Work out the finished part from the listing and answer in its coordinate system (mm). Round coordinates to 2 decimals unless told otherwise and drop trailing zeros. Order: outer loops, then holes, each group sorted by start corner. A loop starts at its lowest first (then second) coordinate and runs counter-clockwise, first axis right, second up. Notation, with made-up numbers: (74.25, -12.75) - (98.25, -12.75) arc R20 cw to (98.25, 0.25) - close; hole circle Ø6 at (60, 71.25). An arc over 180 degrees is marked (long way). One line per question, with ' | ' between items. Start each with the question number.
from build123d import *

# Parameters (mm, degrees)
SKETCH1_R           = 2.5
SKETCH1_R_2         = 2.7
BOSS_EXTRUDE1_DEPTH = 4
SKETCH4_W           = 280
SKETCH4_H           = 240
SKETCH4_W_2         = 250
SKETCH4_H_2         = 210
CUT_EXTRUDE2_DEPTH  = 10
SKETCH5_R           = 2.5
CUT_EXTRUDE3_DEPTH  = 10


with BuildPart() as part:
    # Sketch1 → Boss-Extrude1 (new body)
    with BuildSketch(Plane(origin=(0, 0, 0), x_dir=(1, 0, 0), z_dir=(0, 1, 0))):
        Polygon((-140, 120), (-140, -120), (140, -120), (140, 120), (35, 120), (35, 40), (-40, 40), (-40, 120), align=None)
        with Locations(Location((-116, -92, 0), (0, 0, 270))):
            Circle(SKETCH1_R, mode=Mode.SUBTRACT)
        with BuildLine():
            ThreePointArc((-70, -85), (-72.928932188, -92.071067812), (-80, -95))
            Line((-80, -95), (-105, -95))
            ThreePointArc((-105, -95), (-112.071067812, -92.071067812), (-115, -85))
            Line((-115, -85), (-115, -45))
            ThreePointArc((-115, -45), (-112.071067812, -37.928932188), (-105, -35))
            Line((-105, -35), (-80, -35))
            ThreePointArc((-80, -35), (-72.928932188, -37.928932188), (-70, -45))
            Line((-70, -45), (-70, -85))
        make_face(mode=Mode.SUBTRACT)
        with Locations(Location((-69.5, -95, 0), (0, 0, 270))):
            Circle(SKETCH1_R, mode=Mode.SUBTRACT)
        with Locations(Location((-19.5, -95, 0), (0, 0, 270))):
            Circle(SKETCH1_R, mode=Mode.SUBTRACT)
        with Locations(Location((-46, -90, 0), (0, 0, 270))):
            Circle(SKETCH1_R, mode=Mode.SUBTRACT)
        with Locations(Location((-116, 0, 0), (0, 0, 270))):
            Circle(SKETCH1_R, mode=Mode.SUBTRACT)
        with Locations(Location((-46, -41, 0), (0, 0, 270))):
            Circle(SKETCH1_R, mode=Mode.SUBTRACT)
        with Locations(Location((-58, -25, 0), (0, 0, 270))):
            Circle(SKETCH1_R_2, mode=Mode.SUBTRACT)
        with Locations(Location((17, -95, 0), (0, 0, 270))):
            Circle(SKETCH1_R, mode=Mode.SUBTRACT)
        with Locations(Location((67, -95, 0), (0, 0, 270))):
            Circle(SKETCH1_R, mode=Mode.SUBTRACT)
        with Locations(Location((46, -90, 0), (0, 0, 270))):
            Circle(SKETCH1_R, mode=Mode.SUBTRACT)
        with Locations(Location((116, -92, 0), (0, 0, 270))):
            Circle(SKETCH1_R, mode=Mode.SUBTRACT)
        with BuildLine():
            ThreePointArc((70, -45), (72.928932188, -37.928932188), (80, -35))
            Line((80, -35), (105, -35))
            ThreePointArc((105, -35), (112.071067812, -37.928932188), (115, -45))
            Line((115, -45), (115, -85))
            ThreePointArc((115, -85), (112.071067812, -92.071067812), (105, -95))
            Line((105, -95), (80, -95))
            ThreePointArc((80, -95), (72.928932188, -92.071067812), (70, -85))
            Line((70, -85), (70, -45))
        make_face(mode=Mode.SUBTRACT)
        with Locations(Location((46, -41, 0), (0, 0, 270))):
            Circle(SKETCH1_R, mode=Mode.SUBTRACT)
        with Locations(Location((58, -25, 0), (0, 0, 270))):
            Circle(SKETCH1_R_2, mode=Mode.SUBTRACT)
        with Locations(Location((116, 0, 0), (0, 0, 270))):
            Circle(SKETCH1_R, mode=Mode.SUBTRACT)
        with BuildLine():
            Line((-111.163447186, 65), (-86.163447186, 65))
            ThreePointArc((-86.163447186, 65), (-79.092379374, 62.071067812), (-76.163447186, 55))
            Line((-76.163447186, 55), (-76.163447186, 15))
            ThreePointArc((-76.163447186, 15), (-79.092379374, 7.928932188), (-86.163447186, 5))
            Line((-86.163447186, 5), (-111.163447186, 5))
            ThreePointArc((-111.163447186, 5), (-118.234514998, 7.928932188), (-121.163447186, 15))
            Line((-121.163447186, 15), (-121.163447186, 55))
            ThreePointArc((-121.163447186, 55), (-118.234514998, 62.071067812), (-111.163447186, 65))
        make_face(mode=Mode.SUBTRACT)
        with Locations(Location((-58, 35, 0), (0, 0, 270))):
            Circle(SKETCH1_R_2, mode=Mode.SUBTRACT)
        with Locations(Location((58, 35, 0), (0, 0, 270))):
            Circle(SKETCH1_R_2, mode=Mode.SUBTRACT)
        with BuildLine():
            Line((76.163447186, 15), (76.163447186, 55))
            ThreePointArc((76.163447186, 55), (79.092379374, 62.071067812), (86.163447186, 65))
            Line((86.163447186, 65), (111.163447186, 65))
            ThreePointArc((111.163447186, 65), (118.234514998, 62.071067812), (121.163447186, 55))
            Line((121.163447186, 55), (121.163447186, 15))
            ThreePointArc((121.163447186, 15), (118.234514998, 7.928932188), (111.163447186, 5))
            Line((111.163447186, 5), (86.163447186, 5))
            ThreePointArc((86.163447186, 5), (79.092379374, 7.928932188), (76.163447186, 15))
        make_face(mode=Mode.SUBTRACT)
    extrude(amount=BOSS_EXTRUDE1_DEPTH)

    # Sketch4 → Cut-Extrude2 (cut)
    with BuildSketch(Plane(origin=(0, 4, 0), x_dir=(1, 0, 0), z_dir=(0, 1, 0))):
        Rectangle(SKETCH4_W, SKETCH4_H)
        Rectangle(SKETCH4_W_2, SKETCH4_H_2, mode=Mode.SUBTRACT)
    extrude(amount=-CUT_EXTRUDE2_DEPTH, mode=Mode.SUBTRACT)

    # Sketch5 → Cut-Extrude3 (cut)
    with BuildSketch(Plane(origin=(0, 4, 0), x_dir=(1, 0, 0), z_dir=(0, 1, 0))):
        with Locations(Location((-111.290658089, 73.532159386, 0), (0, 0, 270))):
            Circle(SKETCH5_R)
        with Locations(Location((-57.899945704, 89.235310087, 0), (0, 0, 270))):
            Circle(SKETCH5_R)
        with Locations(Location((53.295143169, 89.235310087, 0), (0, 0, 270))):
            Circle(SKETCH5_R)
        with Locations(Location((106.685855553, 73.532159386, 0), (0, 0, 270))):
            Circle(SKETCH5_R)
        Polygon((-40, 105), (-125, 80), (-125, 105), align=None)
        Polygon((35, 105), (125, 105), (125, 80), align=None)
    extrude(amount=-CUT_EXTRUDE3_DEPTH, mode=Mode.SUBTRACT)


solid = part.part
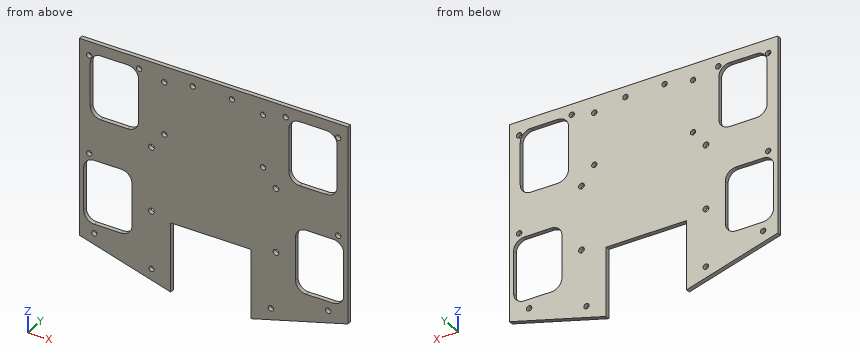
1) Flat-ended cylindrical pins translate along their axes: pin 1 (1.2 mm diameter, centred on x = 96.5, y = 1.5, fed in from -Z); pin 2 (12 mm diameter, centred on x = -2.5, z = -25, fed in from -Y); pin 3 (2 mm diameter, centred on x = -99.5, y = 1.5, fed in from -Z). Find the tip coordinate at first contact, or state that the pin passes through.
2) Straight lines are drawn through the part: line 1 (X direction, y = 1.4, z = -30); line 2 (X direction, y = 0.9, z = 25); line 3 (X direction, y = 1.75, z = -63). For each, find the intervals that lie inside material, in ascending order.
3) Section C-C on x = 9 is taken. Give the vertices of the cut face in (y, z).
4) Section D-D on y = 1.3 is taken. Give the number of separate pieces and of enclosed holes in the cut face, and give its area (3 significant figures).
5) Section B-B on z = 79.5 is taken. Give the vertices of the cut face in (x, y).
6) Section A-A on z = -52 is taken. Give the vertices of the cut face in (x, y).
Recorded:
1) pin 1: stops at z = -88.08 | pin 2: stops at y = 0 | pin 3: stops at z = -87.79
2) line 1: x = -125 to -121.16, -76.16 to 76.16, 121.16 to 125 | line 2: x = -125 to -60.7, -55.3 to 55.3, 60.7 to 125 | line 3: x = -125 to -117.16, -80.16 to -40, 35 to 80.16, 117.16 to 125
3) outline: (0, -40) - (4, -40) - (4, 105) - (0, 105) - close
4) separate pieces: 1 | enclosed holes: 24 | area: 34,600 mm²
5) outline: (-125, 0) - (-115, 0) - (-115, 4) - (-125, 4) - close; (-70, 0) - (70, 0) - (70, 4) - (-70, 4) - close; (115, 0) - (125, 0) - (125, 4) - (115, 4) - close
6) outline: (-125, 0) - (-121.16, 0) - (-121.16, 4) - (-125, 4) - close; (-76.16, 0) - (-40, 0) - (-40, 4) - (-76.16, 4) - close; (35, 0) - (76.16, 0) - (76.16, 4) - (35, 4) - close; (121.16, 0) - (125, 0) - (125, 4) - (121.16, 4) - close
